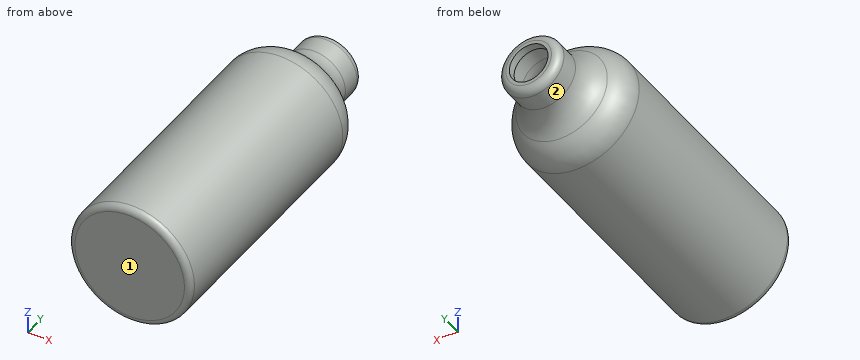
```python
from build123d import *

# Parameters (mm, degrees)
SKETCH2_R          = 7.9375
CUT_EXTRUDE1_DEPTH = 12.7


with BuildPart() as part:
    # Sketch1 → Revolve-Thin2 (revolve)
    with BuildSketch(Plane.XY):
        with BuildLine():
            Line((0, 0), (22.46, 0))
            ThreePointArc((22.46, 0), (24.256051224, 0.743948776), (25, 2.54))
            Line((25, 2.54), (25, 100.324643513))
            ThreePointArc((25, 100.324643513), (23.327352357, 106.624445097), (18.75, 111.264821756))
            ThreePointArc((18.75, 111.264821756), (14.172647643, 115.905198416), (12.5, 122.205))
            Line((12.5, 122.205), (12.5, 129.825))
            ThreePointArc((12.5, 129.825), (11.57006403, 132.07006403), (9.325, 133))
            Line((9.325, 133), (0, 133))
            Line((0, 133), (0, 129.825))
            Line((0, 129.825), (9.325, 129.825))
            Line((9.325, 129.825), (9.325, 122.205))
            ThreePointArc((9.325, 122.205), (11.415809554, 114.33024802), (17.1375, 108.529777196))
            ThreePointArc((17.1375, 108.529777196), (20.570514268, 105.049494701), (21.825, 100.324643513))
            Line((21.825, 100.324643513), (21.825, 3.175))
            Line((21.825, 3.175), (0, 3.175))
            Line((0, 3.175), (0, 0))
        make_face()
    revolve(axis=Axis((0, 133, 0), (0, -1, 0)))

    # Sketch2 → Cut-Extrude1 (cut)
    with BuildSketch(Plane(origin=(0, 133, 0), x_dir=(1, 0, 0), z_dir=(0, 1, 0))):
        Circle(SKETCH2_R)
    extrude(amount=-CUT_EXTRUDE1_DEPTH, mode=Mode.SUBTRACT)


solid = part.part
```
For this review, take the finished solid that the model builds, in its own axes (mm). Face numbers are marked on the shaded views. A direction names the side the tool comes from. Coordinates: 2 decimals unless noted, no trailing zeros. Write each loop counter-clockwise with the first axis right and the second up, starting at its lowest first coordinate (ties: lowest second). Pieces come first, ordered by that corner, then holes. Notation, with made-up numbers: (-14.75, 3) - (8.25, 3) arc R15 cw to (8.25, 31) - close; hole circle Ø10 at (-18.75, 6). An arc over 180 degrees is marked (long way). Answer in a Markdown table with one row per item. Add a question column.
Q1. Tool access review of the marked faces 1 and 2: name each direction out of +Z, -Z, +X, -X, +Y, -Y from which nothing blocks a thin tool from reaching the whole face with its end or side.
Q2. We need section A-A, the plane y = 41.5. State the section outline as (x, z) points (3 decimals), and give its area (3 significant figures).
Q3. For P1, Ø1, axis at x = 4, y = 54.5, coming from the +Z side; P2, Ø8, axis at x = 8, z = 19, coming from the +Y side; P3, Ø1.5, axis at x = 1.5, y = 116.5, coming from the +Z side, all flat-tipped, find the tip position at first contact; note any pin that passes through.
Q4. For probe 1 along Z at (x, y) = (1, 14); probe 2 along Y at (x, z) = (8, -0.5) (3 decimals); probe 3 along Z at (x, y) = (0, 126) (3 decimals), list the stretches that pass through material, from the lowest coordinate up.
Answer list:
| question | item | result |
|---|---|---|
| 1 | face 1 | +Z, -Z, +X, -X, -Y |
| 1 | face 2 | +Y |
| 2 | outline | circle Ø50 at (0, 0); hole circle Ø43.65 at (0, 0) |
| 2 | area | 467 mm2 |
| 3 | P1 | stops at z = 24.75 |
| 3 | P2 | stops at y = 112.85 |
| 3 | P3 | stops at z = 14.19 |
| 4 | probe 1 | z = -24.98 to -21.8, 21.8 to 24.98 |
| 4 | probe 2 | y = 0 to 3.175, 129.825 to 133 |
| 4 | probe 3 | z = -12.5 to -9.325, 9.325 to 12.5 |
